For this review, use the dimensioned drawing (mm, ordinates from the lowest corner) and the shaded views. A direction names the side the tool comes from. Coordinates: 2 decimals unless noted, no trailing zeros. Loops run counter-clockwise (first coordinate to the right, second up) from the corner with the lowest first, then second, coordinate; pieces in that order, holes last.
1. Take a section at B-B, the plane x = 18.25. State the section outline as (y, z) points.
2. Take a section at C-C, the plane y = 3.25. State the section outline as (x, z) points, then the cut area to 3 significant figures.
3. Clearance check with flat-ended pins moving along their axes: P1, Ø3.5, axis at y = 7.5, z = 27.15, coming from the -X side; P2, Ø1.2, axis at x = 27.5, z = 31.5, coming from the -Y side; P3, Ø1.2, axis at x = 27.5, z = 5, coming from the +Y side; P4, Ø10, axis at x = 18.25, z = 18.25, coming from the -Y side (3 decimals). State where each tip first meets the part, or that it passes through.
4. Take a section at A-A, the plane z = 18.25. State the section outline as (x, y) points, then the cut area to 4 significant figures.
5. Mouldability with a two-part tool opening along X and no side actions: class the marked faces 3, 4, 5 and 6 as pulls with the +X half, pulls with the -X half, needs draft (parallel to the pull), parting line crosses it, or undercut.
6. Take a section at D-D, the plane z = 9.35. State the section outline as (x, y) points, then the cut area to 4 significant figures.
7. Machinability: for the marked faces 1 and 2, which of the approach directions +Z, -Z, +X, -X, +Y, -Y give a long, thin tool a straight path to every point of the face, cutting with its end or side? Answer none if there is none.
8. To check wall thickness, follow probe 1 along Z at (x, y) = (27.5, 3.25); probe 2 along X at (y, z) = (12, 26); probe 3 along Y at (x, z) = (1.45, 27.15). State the ranges of each line that lie inside material, in increasing order.
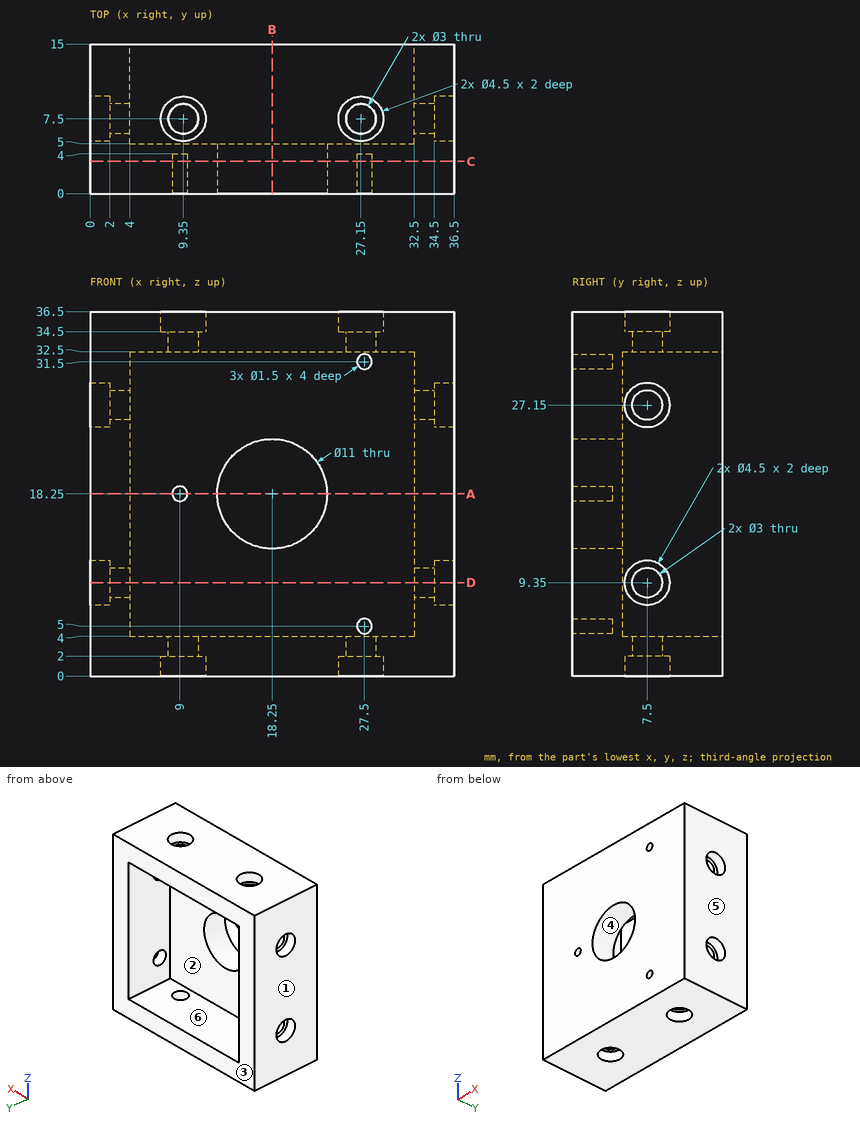
Results list:
1. outline: (0, 0) - (15, 0) - (15, 4) - (5, 4) - (5, 12.75) - (0, 12.75) - close; (0, 23.75) - (5, 23.75) - (5, 32.5) - (15, 32.5) - (15, 36.5) - (0, 36.5) - close
2. outline: (0, 0) - (36.5, 0) - (36.5, 36.5) - (0, 36.5) - close; hole circle Ø1.5 at (9, 18.25); hole circle Ø11 at (18.25, 18.25); hole circle Ø1.5 at (27.5, 5); hole circle Ø1.5 at (27.5, 31.5)
2. area: 1,230 mm2
3. P1: stops at x = 2
3. P2: stops at y = 4
3. P3: stops at y = 5
3. P4: passes through
4. outline: (0, 0) - (8.25, 0) - (8.25, 4) - (9.75, 4) - (9.75, 0) - (12.75, 0) - (12.75, 5) - (4, 5) - (4, 15) - (0, 15) - close; (23.75, 0) - (36.5, 0) - (36.5, 15) - (32.5, 15) - (32.5, 5) - (23.75, 5) - close
4. area: 201.5 mm2
5. face 3: needs draft
5. face 4: undercut
5. face 5: pulls with the +X half
5. face 6: undercut
6. outline: (0, 0) - (36.5, 0) - (36.5, 5.25) - (34.5, 5.25) - (34.5, 6) - (32.5, 6) - (32.5, 5) - (4, 5) - (4, 6) - (2, 6) - (2, 5.25) - (0, 5.25) - close; (0, 9.75) - (2, 9.75) - (2, 9) - (4, 9) - (4, 15) - (0, 15) - close; (32.5, 9) - (34.5, 9) - (34.5, 9.75) - (36.5, 9.75) - (36.5, 15) - (32.5, 15) - close
6. area: 232.5 mm2
7. face 1: +Z, -Z, -X, +Y, -Y
7. face 2: +Y
8. probe 1: z = 0 to 4.25, 5.75 to 30.75, 32.25 to 36.5
8. probe 2: x = 0 to 4, 32.5 to 36.5
8. probe 3: y = 0 to 5.25, 9.75 to 15
